```python
from build123d import *

# Parameters (mm, degrees)
SKETCH1_R           = 4.7625
SKETCH1_R_2         = 2.159
SKETCH1_R_3         = 1.1303
BOSS_EXTRUDE1_DEPTH = 1.7145
SKETCH2_W           = 3.81
SKETCH2_H           = 2.54
CUT_EXTRUDE1_DEPTH  = 1.7145
SKETCH3_W           = 41.91
SKETCH3_H           = 9.525
CUT_EXTRUDE2_DEPTH  = 1.7145
FILLET1_R           = 0.762


with BuildPart() as part:
    # Sketch1 → Boss-Extrude1 (new body)
    with BuildSketch(Plane.XY):
        with BuildLine():
            Line((-33.613, 9.245), (33.613, 9.245))
            Line((33.613, 9.245), (33.613, 34.01))
            Line((33.613, 34.01), (0, 34.01))
            ThreePointArc((0, 34.01), (-16.098329106, 29.958703243), (-28.361368091, 18.77))
            Line((-28.361368091, 18.77), (-33.613, 18.77))
            Line((-33.613, 18.77), (-33.613, 9.245))
        make_face()
        with Locations((26.852588835, 27.025)):
            Circle(SKETCH1_R, mode=Mode.SUBTRACT)
        with Locations((-25.6374, 14.5155)):
            Circle(SKETCH1_R_2, mode=Mode.SUBTRACT)
        with Locations((28.8886, 14.5155)):
            Circle(SKETCH1_R_2, mode=Mode.SUBTRACT)
        with Locations((30.662588835, 20.675)):
            Circle(SKETCH1_R_3, mode=Mode.SUBTRACT)
        with Locations((16.692588835, 29.565)):
            Circle(SKETCH1_R_3, mode=Mode.SUBTRACT)
    extrude(amount=BOSS_EXTRUDE1_DEPTH)

    # Sketch2 → Cut-Extrude1 (cut)
    with BuildSketch(Plane.XY.offset(1.7145)):
        with Locations((-1.644140797, 29.166672544)):
            Rectangle(SKETCH2_W, SKETCH2_H)
        with Locations((-1.644140797, 24.086672544)):
            Rectangle(SKETCH2_W, SKETCH2_H)
    extrude(amount=-CUT_EXTRUDE1_DEPTH, mode=Mode.SUBTRACT)

    # Sketch3 → Cut-Extrude2 (cut)
    with BuildSketch(Plane.XY.offset(1.7145)):
        with Locations((0, 14.0075)):
            Rectangle(SKETCH3_W, SKETCH3_H)
    extrude(amount=-CUT_EXTRUDE2_DEPTH, mode=Mode.SUBTRACT)

    # Fillet1
    fillet1_edges = [part.edges().sort_by_distance(p)[0] for p in [
        (-28.361368091, 18.77, 0.85725),
        (33.613, 34.01, 0.85725),
        (33.613, 9.245, 0.85725),
        (-33.613, 9.245, 0.85725),
        (-33.613, 18.77, 0.85725),
        (-20.955, 9.245, 0.85725),
        (20.955, 9.245, 0.85725),
    ]]
    fillet(fillet1_edges, radius=FILLET1_R)


solid = part.part
```
Geometry: final body of the model. Coordinates: model frame, mm. A direction names the side the tool comes from. Round coordinates to 2 decimals unless told otherwise and drop trailing zeros. Order: outer loops, then holes, each group sorted by start corner. A loop starts at its lowest first (then second) coordinate and runs counter-clockwise, first axis right, second up. Notation, with made-up numbers: (73, 41) - (131, 41) arc R17 cw to (131, 59) - close; hole circle Ø5 at (35, -0.5). An arc over 180 degrees is marked (long way). Use CSV: the item, a comma, the result in double quotes. Start each with the question number.
Q1. Mould query, pull axis X, two halves, no side actions, for faces 1 (the face through (0, 18.77, 1)), 2 (the face through (17, 34.01, 1)), 3 (the face through (-33.613, 14, 1)). Classes: +X half, -X half, draft (parallel to the pull), parting line (faces both ways), or undercut.
Q2. Section query C-C (y = 16). Return loops of the section in (x, z) (1 decimal), and give its area (3 significant figures).
Q3. Section query A-A (y = 11). Return loops of the section in (x, z) (1 decimal), and give its area (3 significant figures).
Q4. Section query B-B (x = 16.5). Return loops of the section in (y, z).
Q5. Material intervals for line 1 along X through (y, z) = (25, 0.3); line 2 along X through (y, z) = (18, 0.25) (3 decimals); line 3 along Y through (x, z) = (26.5, 1) (3 decimals), sorted ascending. Write a range as from..to.
Q6. Section query D-D (z = 1.25). State how many separate pieces and enclosed holes the cut face has, and give its area (3 significant figures).
Q7. Access query for faces 4 (the face through (-31, 18.77, 1)), 5 (the face through (-3.549, 29, 1)), 6 (the face through (-20.955, 14, 1)). Directions: +Z, -Z, +X, -X, +Y, -Y. A direction counts if a zero-diameter tool reaches every point of the face in a straight line with its end or side. Return the directions, or none.
Q8. First-contact query: pin 1 (7 mm diameter, centred on x = -25.64, y = 14.52, fed in from +Z); pin 2 (0.5 mm diameter, centred on x = -2.5, z = 0.5, fed in from -Y); pin 3 (2.5 mm diameter, centred on x = 28.89, y = 14.52, fed in from -Z); pin 4 (0.5 mm diameter, centred on y = 30, z = 0.5, fed in from -X). Flat tips, straight axial feed; report the tip coordinate or a pass-through.
Result set:
1,face 1,"undercut"
1,face 2,"draft"
1,face 3,"-X half"
2,outline,"(-33.6, 0) - (-27.2, 0) - (-27.2, 1.7) - (-33.6, 1.7) - close; (-24.1, 0) - (-21, 0) - (-21, 1.7) - (-24.1, 1.7) - close; (21, 0) - (27.3, 0) - (27.3, 1.7) - (21, 1.7) - close; (30.5, 0) - (33.6, 0) - (33.6, 1.7) - (30.5, 1.7) - close"
2,area,"32.7 mm2"
3,outline,"(-33.6, 0) - (-21, 0) - (-21, 1.7) - (-33.6, 1.7) - close; (21, 0) - (33.6, 0) - (33.6, 1.7) - (21, 1.7) - close"
3,area,"43.4 mm2"
4,outline,"(18.77, 0) - (28.45, 0) - (28.45, 1.71) - (18.77, 1.71) - close; (30.68, 0) - (34.01, 0) - (34.01, 1.71) - (30.68, 1.71) - close"
5,line 1,"x = -23.06..-3.55, 0.26..22.54, 31.16..33.61"
5,line 2,"x = -33.613..-20.955, 20.955..33.613"
5,line 3,"y = 9.245..22.276, 31.774..34.01"
6,separate pieces,"1"
6,enclosed holes,"7"
6,area,"929 mm2"
7,face 4,"+Z, -Z, -X, +Y"
7,face 5,"+Z, -Z"
7,face 6,"+Z, -Z, -Y"
8,pin 1,"stops at z = 1.71"
8,pin 2,"stops at y = 18.77"
8,pin 3,"passes through"
8,pin 4,"stops at x = -16.48"
